```python
from build123d import *

# Parameters (mm, degrees)
SKETCH1_W           = 25
SKETCH1_H           = 10
SKETCH1_R           = 1.15
BOSS_EXTRUDE1_DEPTH = 3
SKETCH3_W           = 8
SKETCH3_H           = 18
SKETCH3_R           = 0.7
BOSS_EXTRUDE2_DEPTH = 10
SKETCH5_R           = 0.975
CUT_EXTRUDE2_DEPTH  = 3.5
CHAMFER1_SIZE       = 3


with BuildPart() as part:
    # Sketch1 → Boss-Extrude1 (new body)
    with BuildSketch(Plane(origin=(0, 0, 0), x_dir=(1, 0, 0), z_dir=(0, 1, 0))):
        Rectangle(SKETCH1_W, SKETCH1_H)
        with Locations(Location((-10, 2.5, 0), (0, 0, 270))):
            Circle(SKETCH1_R, mode=Mode.SUBTRACT)
        with Locations(Location((-10, -2.5, 0), (0, 0, 270))):
            Circle(SKETCH1_R, mode=Mode.SUBTRACT)
        with Locations(Location((10, 2.5, 0), (0, 0, 270))):
            Circle(SKETCH1_R, mode=Mode.SUBTRACT)
        with Locations(Location((10, -2.5, 0), (0, 0, 270))):
            Circle(SKETCH1_R, mode=Mode.SUBTRACT)
    extrude(amount=BOSS_EXTRUDE1_DEPTH)

    # Sketch3 → Boss-Extrude2 (add)
    with BuildSketch(Plane(origin=(0, 0, -5), x_dir=(-1, 0, 0), z_dir=(0, 0, -1))):
        with Locations((0, 9)):
            Rectangle(SKETCH3_W, SKETCH3_H)
        with Locations((0, 14)):
            Circle(SKETCH3_R, mode=Mode.SUBTRACT)
    extrude(amount=-BOSS_EXTRUDE2_DEPTH)

    # Sketch5 → Cut-Extrude2 (cut)
    with BuildSketch(Plane(origin=(0, 18, 0), x_dir=(1, 0, 0), z_dir=(0, 1, 0))):
        with Locations(Location((0, 3, 0), (0, 0, 180))):
            Circle(SKETCH5_R)
        with Locations(Location((0, -3, 0), (0, 0, 180))):
            Circle(SKETCH5_R)
    extrude(amount=-CUT_EXTRUDE2_DEPTH, mode=Mode.SUBTRACT)

    # Chamfer1
    chamfer1_edges = [part.edges().sort_by_distance(p)[0] for p in [
        (-4, 3, 0),
        (4, 3, 0),
    ]]
    chamfer(chamfer1_edges, length=CHAMFER1_SIZE)


solid = part.part
```
For this review, take the finished solid that the model builds, in its own axes (mm). A direction names the side the tool comes from. Round coordinates to 2 decimals unless told otherwise and drop trailing zeros. Write each loop counter-clockwise with the first axis right and the second up, starting at its lowest first coordinate (ties: lowest second). Pieces come first, ordered by that corner, then holes. Notation, with made-up numbers: (-33, -30.75) - (16, -30.75) arc R34 ccw to (16, 6.25) - close; hole circle Ø7 at (23, 22). An arc over 180 degrees is marked (long way). Put each result on its own line as item: value.
Q1. We need section D-D (x = 10). Give the boundary of the cut face in (y, z), and give its area (3 significant figures).
Solved:
outline: (0, -5) - (3, -5) - (3, -3.65) - (0, -3.65) - close; (0, -1.35) - (3, -1.35) - (3, 1.35) - (0, 1.35) - close; (0, 3.65) - (3, 3.65) - (3, 5) - (0, 5) - close
area: 16.2 mm2
Q2. We need section B-B (y = 14). Give the boundary of the cut face in (x, z), and give its area (3 significant figures).
Solved:
outline: (-4, -5) - (-0.7, -5) - (-0.7, 5) - (-4, 5) - close; (0.7, -5) - (4, -5) - (4, 5) - (0.7, 5) - close
area: 66.0 mm2
Q3. We need section A-A (z = 1). Give the boundary of the cut face in (x, y), and give its area (3 significant figures).
Solved:
outline: (-12.5, 0) - (12.5, 0) - (12.5, 3) - (7, 3) - (4, 6) - (4, 18) - (-4, 18) - (-4, 6) - (-7, 3) - (-12.5, 3) - close; hole circle Ø1.4 at (0, 14)
area: 202 mm2
Q4. Machinability: for faces 1 (the face through (-4, 12, 0)), 2 (the face through (0.127, 16.274, 3.967)), 3 (the face through (-11.02, 1.48, 3.03)), 4 (the face through (10, 3, 0)), which of the approach directions +Z, -Z, +X, -X, +Y, -Y give a long, thin tool a straight path to every point of the face, cutting with its end or side? Answer none if there is none.
Solved:
face 1: +Z, -Z, -X, +Y
face 2: +Y
face 3: +Y, -Y
face 4: +Z, -Z, +X, +Y
Q5. Mouldability with a two-part tool opening along Z and no side actions: class faces 5 (the face through (-12.5, 1, 0)), 6 (the face through (0, 7, 5)), 7 (the face through (8.98, 1.48, 3.03)) as released by +Z, released by -Z, zero draft, split by the parting line, or undercut.
Solved:
face 5: zero draft
face 6: released by +Z
face 7: undercut
Q6. Wall thickness on probe 1 along Z at (x, y) = (0, 16.1) (3 decimals); probe 2 along Y at (x, z) = (0, 0.25); probe 3 along X at (y, z) = (1.9, 2.5): over which ranges is each line inside the solid? List them lowest first.
Solved:
probe 1: z = -5 to -3.975, -2.025 to 2.025, 3.975 to 5
probe 2: y = 0 to 13.3, 14.7 to 18
probe 3: x = -12.5 to -11.15, -8.85 to 8.85, 11.15 to 12.5
Q7. Insertion check: pin 1 Ø0.5 at (x, z) = (0.5, -3) entering from +Y; pin 2 Ø5 at (y, z) = (7, -4) entering from -X; pin 3 Ø6 at (x, z) = (-9.5, -2) entering from +Y; pin 4 Ø1.1 at (x, y) = (0, 14) entering from +Z. Each pin has a flat end and moves straight along its axis. Give the tip position at first contact, or say it passes through.
Solved:
pin 1: stops at y = 14.5
pin 2: stops at x = -5.5
pin 3: stops at y = 3.5
pin 4: passes through
Q8. We need section C-C (z = -1.75). Give the boundary of the cut face in (x, y), and give its area (3 significant figures).
Solved:
outline: (-12.5, 0) - (-10.87, 0) - (-10.87, 3) - (-12.5, 3) - close; (-9.13, 0) - (9.13, 0) - (9.13, 3) - (7, 3) - (4, 6) - (4, 18) - (-4, 18) - (-4, 6) - (-7, 3) - (-9.13, 3) - close; (10.87, 0) - (12.5, 0) - (12.5, 3) - (10.87, 3) - close; hole circle Ø1.4 at (0, 14)
area: 192 mm2
